Build history of the part. All positions in model axes, mm. Round coordinates to 2 decimals unless told otherwise and drop trailing zeros. Order: outer loops, then holes, each group sorted by start corner. A loop starts at its lowest first (then second) coordinate and runs counter-clockwise, first axis right, second up. Notation, with made-up numbers: (42.5, 48.5) -> (89.5, 48.5) arc R11 ccw to (89.5, 66.5) -> close; hole circle Ø2 at (-26.75, -39.75). An arc over 180 degrees is marked (long way). Answer as a JSON object with one key per item and string values.
from build123d import *

# Parameters (mm, degrees)
F2_DEPTH = 25.4
F0_R     = 45.389454
F3_DEPTH = 25.4


with BuildPart() as f2:
    # F1 (on face) → F2 (new body)
    with BuildSketch(Plane.XZ):
        with BuildLine():
            ThreePointArc((-408.650134, -138.321041), (-500.899934, 120.173805), (-237.660617, 197.856963))
            ThreePointArc((-237.660617, 197.856963), (-797.702842, 271.136049), (-408.650134, -138.321041))
        make_face()
    extrude(amount=F2_DEPTH)

    # F0 (on Front) → F3 (join)
    with BuildSketch(Plane.XZ):
        with BuildLine():
            ThreePointArc((88.884516, -22.918433), (79.660927, 15.310849), (118.946802, 17.092003))
            ThreePointArc((118.946802, 17.092003), (153.828866, 94.879416), (165.768481, 179.289639))
            ThreePointArc((165.768481, 179.289639), (-423.061654, 287.455309), (88.884516, -22.918433))
        make_face()
        Circle(F0_R, mode=Mode.SUBTRACT)
    extrude(amount=F3_DEPTH)


solid = f2.part
1) Cut at C-C, the plane y = -11.25. Give the cut face in (x, z).
Checked values:
{"outline": "(-442.81, 187.9) arc R304.35 ccw to (88.88, -22.92) arc R25.49 cw (long way) to (118.95, 17.09) arc R304.35 ccw to (165.77, 179.29) arc R304.35 ccw to (-363.72, 384.09) arc R299.6 ccw (long way) to (-408.65, -138.32) arc R188.88 cw to start; hole circle Ø90.78 at (0, 0)"}
2) Cut at A-A, the plane z = 408.5. Give the cut face in (x, y), plus the area to 3 significant figures.
Checked values:
{"outline": "(-653.66, -25.4) -> (-407.66, -25.4) -> (-407.66, 0) -> (-653.66, 0) -> close; (-338.81, -25.4) -> (61.65, -25.4) -> (61.65, 0) -> (-338.81, 0) -> close", "area": "16,400 mm²"}
3) Pull direction X, two halves, no side cores. Call faces 1 (the face through (-339, 0, 164)), 2 (the face through (43.293, -12.522, 13.634)), 3 (the face through (79.289, -12.522, 14.804)): pulls with the +X half, pulls with the -X half, needs draft (parallel to the pull), parting line crosses it, or undercut.
Checked values:
{"face 1": "needs draft", "face 2": "undercut", "face 3": "undercut"}
4) Cut at B-B, the plane x = 0. Give the cut face in (y, z), plus the area to 3 significant figures.
Checked values:
{"outline": "(-25.4, -91.68) -> (0, -91.68) -> (0, -45.39) -> (-25.4, -45.39) -> close; (-25.4, 45.39) -> (0, 45.39) -> (0, 450.26) -> (-25.4, 450.26) -> close", "area": "11,500 mm²"}
5) Flat gauge pins, fed straight in: pin 1 Ø1.5 at (x, z) = (-215.5, 298.5) entering from +Y; pin 2 Ø8 at (x, y) = (-640, -9) entering from -Z; pin 3 Ø10 at (y, z) = (-20.5, -61.5) entering from +X; pin 4 Ø3 at (x, y) = (10.5, -6.5) entering from -Z. Where does each tip first touch, or does it go through?
Checked values:
{"pin 1": "stops at y = 0", "pin 2": "stops at z = -145.16", "pin 3": "stops at x = 53.86", "pin 4": "stops at z = -86.88"}
6) Cut at D-D, the plane z = 0. Give the cut face in (x, y).
Checked values:
{"outline": "(-797.96, -25.4) -> (-518.24, -25.4) -> (-518.24, 0) -> (-797.96, 0) -> close; (-384.52, -25.4) -> (-45.39, -25.4) -> (-45.39, 0) -> (-384.52, 0) -> close; (45.39, -25.4) -> (74.55, -25.4) -> (74.55, 0) -> (45.39, 0) -> close"}
7) Probe L1, parallel to X at y = -17.5, z = -22; L2, parallel to Z at x = -27, y = -15.5; L3, parallel to X at y = -11.75, z = 134. List the from-to ranges inside material, lowest first. Write a range as from..to.
Checked values:
{"L1": "x = -785.64..-512.76, -366.86..-39.7, 39.7..87.17", "L2": "z = -103.87..-36.49, 36.49..462.45", "L3": "x = -830.26..-493.12, -439.54..162.38"}
